Can you work these out from the model? Positions are in its coordinate system, mm. Face numbers are marked on the shaded views. A direction names the side the tool comes from. Coordinates: 2 decimals unless noted, no trailing zeros. Loops run counter-clockwise (first coordinate to the right, second up) from the corner with the lowest first, then second, coordinate; pieces in that order, holes last.
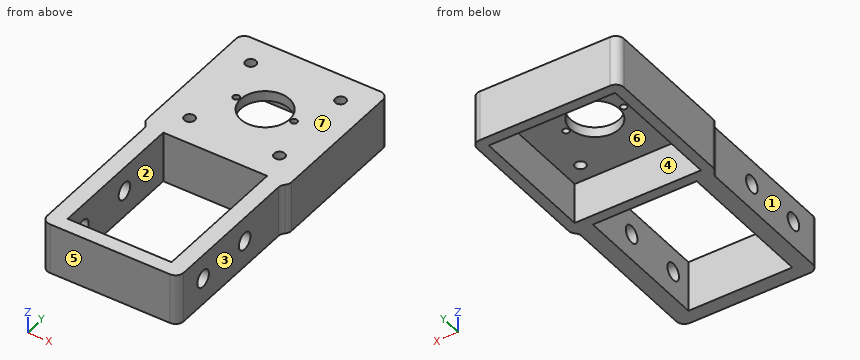
```python
from build123d import *

# Parameters (mm, degrees)
SKETCH1_W                = 39.37
SKETCH1_H                = 39.37
SKETCH1_R                = 1.651
SKETCH1_R_2              = 7.62
SKETCH1_R_3              = 1.016
BOSS_EXTRUDE1_DEPTH      = 3.175
BOSS_EXTRUDE2_DEPTH      = 12.7
BOSS_EXTRUDE2_DEPTH_BACK = 3.175
SKETCH3_W                = 45.72
SKETCH3_H                = 45.72
SKETCH3_W_2              = 39.37
SKETCH3_H_2              = 39.37
SKETCH5_W                = 5.08
SKETCH5_H                = 15.875
BOSS_EXTRUDE3_DEPTH      = 48.26
SKETCH6_W                = 42.545
SKETCH6_H                = 15.875
BOSS_EXTRUDE4_DEPTH      = 4.445
SKETCH7_R                = 2.667
CUT_EXTRUDE1_DEPTH       = 70.979765826
FILLET1_R                = 2.54
FILLET2_R                = 2.54
FILLET3_R                = 2.54


with BuildPart() as part:
    # Sketch1 → Boss-Extrude1 (new body)
    with BuildSketch(Plane.XY):
        with Locations((-19.685, 19.685)):
            Rectangle(SKETCH1_W, SKETCH1_H)
        with Locations((-33.68548, 5.68452)):
            Circle(SKETCH1_R, mode=Mode.SUBTRACT)
        with Locations((-33.68548, 33.68548)):
            Circle(SKETCH1_R, mode=Mode.SUBTRACT)
        with Locations((-5.68452, 5.68452)):
            Circle(SKETCH1_R, mode=Mode.SUBTRACT)
        with Locations((-5.68452, 33.68548)):
            Circle(SKETCH1_R, mode=Mode.SUBTRACT)
        with Locations((-19.685, 19.685)):
            Circle(SKETCH1_R_2, mode=Mode.SUBTRACT)
        with Locations((-28.68549, 19.685)):
            Circle(SKETCH1_R_3, mode=Mode.SUBTRACT)
        with Locations((-10.68451, 19.685)):
            Circle(SKETCH1_R_3, mode=Mode.SUBTRACT)
    extrude(amount=BOSS_EXTRUDE1_DEPTH)

    # Sketch3 → Boss-Extrude2 (add, two sides: drawn at the far end of the back side and taken through both)
    with BuildSketch(Plane(origin=(0, 0, 0), x_dir=(-1, 0, 0), z_dir=(0, 0, -1)).offset(-BOSS_EXTRUDE2_DEPTH_BACK)):
        with Locations((19.685, 19.685)):
            Rectangle(SKETCH3_W, SKETCH3_H)
        with Locations((19.685, 19.685)):
            Rectangle(SKETCH3_W_2, SKETCH3_H_2, mode=Mode.SUBTRACT)
    extrude(amount=BOSS_EXTRUDE2_DEPTH + BOSS_EXTRUDE2_DEPTH_BACK)

    # Sketch5 → Boss-Extrude3 (add)
    with BuildSketch(Plane(origin=(0, -3.175, 0), x_dir=(-1, 0, 0), z_dir=(0, -1, 0))):
        with Locations((38.4175, 4.7625)):
            Rectangle(SKETCH5_W, SKETCH5_H)
        with Locations((0.9525, 4.7625)):
            Rectangle(SKETCH5_W, SKETCH5_H)
    extrude(amount=BOSS_EXTRUDE3_DEPTH)

    # Sketch6 → Boss-Extrude4 (add)
    with BuildSketch(Plane(origin=(-35.8775, -51.435, -12.7), x_dir=(1, 0, 0), z_dir=(0, 1, 0))):
        with Locations((16.1925, -7.9375)):
            Rectangle(SKETCH6_W, SKETCH6_H)
    extrude(amount=BOSS_EXTRUDE4_DEPTH)

    # Sketch7 → Cut-Extrude1 (cut, through all)
    with BuildSketch(Plane.ZY.offset(42.545)):
        with Locations(Location((-4.445, -40.005, 0), (0, 0, 90))):
            Circle(SKETCH7_R)
        with Locations(Location((-4.445, -20.955, 0), (0, 0, 90))):
            Circle(SKETCH7_R)
    extrude(amount=-CUT_EXTRUDE1_DEPTH, mode=Mode.SUBTRACT)

    # Fillet1
    # the kernel refuses this fillet: 2.54 mm, written as the material it adds along each edge
    with BuildSketch(Plane(origin=(1.5875, -3.175, 3.175), x_dir=(1, 0, 0), z_dir=(0, 0, -1))) as fillet1_piece_1:
        with BuildLine():
            CenterArc((2.54, 2.35464302), FILLET1_R, 180, 67.975687163)
            Line((0, 2.35464302), (0, 0))
            Line((0, 0), (1.5875, 0))
        make_face()
    extrude(amount=15.875)
    # the kernel refuses this fillet: 2.54 mm, written as the material it takes off along each edge
    with BuildSketch(Plane(origin=(-40.9575, -51.435, -19.05), x_dir=(1, 0, 0), z_dir=(0, 0, 1))) as fillet1_2_piece_1:
        with BuildLine():
            CenterArc((FILLET1_R, FILLET1_R), FILLET1_R, 180, 90)
            Line((0, FILLET1_R), (0, 0))
            Line((0, 0), (FILLET1_R, 0))
        make_face()
    extrude(amount=28.575, mode=Mode.SUBTRACT)
    with BuildSketch(Plane(origin=(1.5875, -51.435, 9.525), x_dir=(0, 1, 0), z_dir=(0, 0, -1))) as fillet1_2_piece_2:
        with BuildLine():
            CenterArc((FILLET1_R, -FILLET1_R), FILLET1_R, 90, 90)
            Line((0, -FILLET1_R), (0, 0))
            Line((0, 0), (FILLET1_R, 0))
        make_face()
    extrude(amount=28.575, mode=Mode.SUBTRACT)

    # Fillet2
    # the kernel refuses this fillet: 2.54 mm, written as the material it takes off along each edge
    with BuildSketch(Plane(origin=(-42.545, -3.175, 9.061607549), x_dir=(1, 0, 0), z_dir=(0, 0, -1))) as fillet2_piece_1:
        with BuildLine():
            CenterArc((2.54, -2.35464302), FILLET2_R, 112.024312837, 67.975687163)
            Line((0, -2.35464302), (-0.0508, -2.35464302))
            Line((-0.0508, -2.35464302), (-0.0508, 0))
            Line((-0.0508, 0), (0, 0.0508))
            ThreePointArc((0, 0.0508), (0.79375, 0.0508), (1.56845, 0.04709286))
            Line((1.56845, 0.04709286), (1.5875, 0))
        make_face()
    extrude(amount=27.648215098, mode=Mode.SUBTRACT)
    with BuildSketch(Plane(origin=(3.175, 42.545, -19.05), x_dir=(0, -1, 0), z_dir=(0, 0, 1))) as fillet2_piece_2:
        with BuildLine():
            CenterArc((FILLET2_R, -FILLET2_R), FILLET2_R, 90, 90)
            Line((0, -FILLET2_R), (-FILLET2_R * 0.02, -FILLET2_R))
            Line((-FILLET2_R * 0.02, -FILLET2_R), (-FILLET2_R * 0.02, FILLET2_R * 0.02))
            Line((-FILLET2_R * 0.02, FILLET2_R * 0.02), (FILLET2_R, FILLET2_R * 0.02))
            Line((FILLET2_R, FILLET2_R * 0.02), (FILLET2_R, 0))
        make_face()
    extrude(amount=28.575, mode=Mode.SUBTRACT)
    with BuildSketch(Plane(origin=(-42.545, 42.545, 9.525), x_dir=(1, 0, 0), z_dir=(0, 0, -1))) as fillet2_piece_3:
        with BuildLine():
            CenterArc((FILLET2_R, FILLET2_R), FILLET2_R, 180, 90)
            Line((0, FILLET2_R), (-FILLET2_R * 0.02, FILLET2_R))
            Line((-FILLET2_R * 0.02, FILLET2_R), (-FILLET2_R * 0.02, -FILLET2_R * 0.02))
            Line((-FILLET2_R * 0.02, -FILLET2_R * 0.02), (FILLET2_R, -FILLET2_R * 0.02))
            Line((FILLET2_R, -FILLET2_R * 0.02), (FILLET2_R, 0))
        make_face()
    extrude(amount=28.575, mode=Mode.SUBTRACT)
    with BuildSketch(Plane(origin=(3.175, -3.175, -16.035934044), x_dir=(-0.8412426627142054, -0.5406577313139188, 0), z_dir=(0, 0, 1))) as fillet2_piece_4:
        with BuildLine():
            CenterArc((1.41531695, -2.495802653), FILLET2_R, 100.70411186, 46.567463442)
            Line((-0.721439413, -1.122532015), (-0.76417454, -1.095066602))
            Line((-0.76417454, -1.095066602), (-0.042735127, 0.027465413))
            Line((-0.042735127, 0.027465413), (0.009435446, 0.049916053))
            ThreePointArc((0.009435446, 0.049916053), (0.471772317, 0.006602653), (0.934109187, 0.049916053))
            Line((0.934109187, 0.049916053), (0.943544634, 0))
        make_face()
    extrude(amount=22.546868088, mode=Mode.SUBTRACT)

    # Fillet3
    fillet3_edges = [part.edges().sort_by_distance(p)[0] for p in [
        (-40.9575, -3.175, -4.7625),
    ]]
    fillet(fillet3_edges, radius=FILLET3_R)


solid = part.part
```
(1) I want a section at A-A on z = -11. Write out the boundary of the cut face in (x, y) (1 decimal), then the cut area to 3 significant figures.
Check values:
outline: (-42.5, -0.8) arc R2.5 ccw to (-41.8, -2.7) arc R2.5 cw to (-41, -4.5) - (-41, -48.9) arc R2.5 ccw to (-38.4, -51.4) - (-1, -51.4) arc R2.5 ccw to (1.6, -48.9) - (1.6, -5.5) arc R2.5 cw to (2.4, -3.7) arc R2.5 ccw to (3.2, -1.8) - (3.2, 40) arc R2.5 ccw to (0.6, 42.5) - (-40, 42.5) arc R2.5 ccw to (-42.5, 40) - close; hole (-39.4, 0) - (0, 0) - (0, 39.4) - (-39.4, 39.4) - close; hole (-35.9, -47) - (-3.5, -47) - (-3.5, -3.2) - (-35.9, -3.2) - close
area: 1,170 mm2
(2) I want a section at B-B on x = -33.5. Write out the boundary of the cut face in (y, z) (3 decimals).
Check values:
outline: (-51.435, -12.7) - (-46.99, -12.7) - (-46.99, 3.175) - (-51.435, 3.175) - close; (-3.175, -12.7) - (0, -12.7) - (0, 0) - (4.044, 0) - (4.044, 3.175) - (-3.175, 3.175) - close; (7.325, 0) - (32.045, 0) - (32.045, 3.175) - (7.325, 3.175) - close; (35.326, 0) - (39.37, 0) - (39.37, -12.7) - (42.545, -12.7) - (42.545, 3.175) - (35.326, 3.175) - close
(3) I'm going to push flat-ended pins straight in: pin 1 (8.5 mm diameter, centred on y = -40.005, z = -4.445, fed in from -X); pin 2 (2 mm diameter, centred on x = -22.5, y = 26, fed in from -Z); pin 3 (5 mm diameter, centred on y = -29, z = -8, fed in from +X). Where does each tip first touch, or does it pass through?
Check values:
pin 1: stops at x = -40.96
pin 2: stops at z = 0
pin 3: stops at x = 1.59
(4) If I drill on probe 1 along Y at (x, z) = (-9, -5.5) (3 decimals); probe 2 along X at (y, z) = (-13.5, -11.25); probe 3 along X at (y, z) = (30.5, -12) (3 decimals), over which ranges is the centre line in solid material (lowest first)?
Check values:
probe 1: y = -51.435 to -46.99, -3.175 to 0, 39.37 to 42.545
probe 2: x = -40.96 to -35.88, -3.49 to 1.59
probe 3: x = -42.545 to -39.37, 0 to 3.175
(5) Which directions (+Z, -Z, +X, -X, +Y, -Y) give clear straight access to the entire face, cutting with the end or side of a thin tool? Please do the marked faces 1, 2, 3 and 4.
Check values:
face 1: +Z, -Z, -X, -Y
face 2: +Z, -Z
face 3: +Z, -Z, +X, -Y
face 4: -Z
(6) If we mould it in two halves opening along Y, with no side actions, what happens to the marked faces 5, 6 and 7? For each: released by +Y, released by -Y, zero draft, split by the parting line, or undercut.
Check values:
face 5: released by -Y
face 6: undercut
face 7: zero draft
(7) I want a section at D-D on y = 13.5. Write out the boundary of the cut face in (x, z) (3 decimals).
Check values:
outline: (-42.545, -12.7) - (-39.37, -12.7) - (-39.37, 0) - (-24.136, 0) - (-24.136, 3.175) - (-42.545, 3.175) - close; (-15.234, 0) - (0, 0) - (0, -12.7) - (3.175, -12.7) - (3.175, 3.175) - (-15.234, 3.175) - close
(8) I want a section at C-C on y = 31. Write out the boundary of the cut face in (x, z) (3 decimals), then the cut area to 3 significant figures.
Check values:
outline: (-42.545, -12.7) - (-39.37, -12.7) - (-39.37, 0) - (0, 0) - (0, -12.7) - (3.175, -12.7) - (3.175, 3.175) - (-42.545, 3.175) - close
area: 226 mm2
